Could you check a few things on this model? Use its own coordinates, in mm. A direction names the side the tool comes from. Round coordinates to 2 decimals unless told otherwise and drop trailing zeros. Write each loop counter-clockwise with the first axis right and the second up, starting at its lowest first coordinate (ties: lowest second). Pieces come first, ordered by that corner, then holes. Notation, with made-up numbers: M -33.75,-11.5 L -23.75,-11.5 A18 cw -23.75,16.5 Z; hole C 42.25,74.25 d6. An arc over 180 degrees is marked long. One line per item, written item: value. Start each with the question number.
(1) If I drill on L1, parallel to Y at x = 5.5, z = 5 (3 decimals); L2, parallel to X at y = -8.5, z = 10; L3, parallel to X at y = -4.25, z = -11, over which ranges is the centre line in solid material (lowest first)?
(2) Thinking about a two-plate mould opening in X: for faces 5 (the face through (0, -0.025, 19)), 6 (the face through (-13.157, -6, -22)), 7 (the face through (0, -3, 22.542)), 8 (the face through (0, -4.267, 22)), which applies, released by +X, released by -X, zero draft, split by the parting line, or undercut?
(3) I want a section at A-A on z = 8. Please give me the cut outline in (x, y) (1 decimal).
(4) Which directions (+Z, -Z, +X, -X, +Y, -Y) give clear straight access to the entire face, cutting with the end or side of a thin tool? Please do faces 1 (the face through (-5.4, -6.528, 21.9)), 2 (the face through (-10, -9.347, 22)), 3 (the face through (5.893, -8, 22)), 4 (the face through (-9, 0.203, -22)).
(5) I want a section at D-D on z = 20. Please give me the cut outline in (x, y), and give its area (3 significant figures).
(6) I want a section at C-C on y = -2.75. Count the separate pieces of the cut face and the enclosed holes in it, and give its area (3 significant figures).
(7) I'm going to push flat-ended pins straight in: pin 1 Ø1.5 at (y, z) = (-6.5, -19.5) entering from -X; pin 2 Ø1 at (x, z) = (1.5, -14.5) entering from -Y; pin 3 Ø5.5 at (y, z) = (-4.5, -19) entering from +X. Where does each tip first touch, or does it pass through?
```python
from build123d import *

# Parameters (mm, degrees)
BOSS_EXTRUDE1_DEPTH = 16.1925
SKETCH2_R           = 1.27
CUT_EXTRUDE1_DEPTH  = 5.08
BOSS_EXTRUDE2_DEPTH = 5.08
BOSS_EXTRUDE3_DEPTH = 1.27


with BuildPart() as part:
    # Sketch1 → Boss-Extrude1 (new body, symmetric)
    with BuildSketch(Plane.XY):
        Polygon((13.208, 0.254), (13.208, -9.398), (5.842, -9.398), (5.842, -6.985), (4.826, -6.985), (4.826, -6.477), (5.842, -6.477), (5.842, -4.318), (-5.842, -4.318), (-5.842, -6.477), (-4.826, -6.477), (-4.826, -6.985), (-5.842, -6.985), (-5.842, -9.398), (-13.208, -9.398), (-13.208, 0.254), (-7.367499011, 0.254), (-6.958302098, 0), (6.958302098, 0), (7.367499011, 0.254), align=None)
    extrude(amount=BOSS_EXTRUDE1_DEPTH, both=True)

    # Sketch2 → Cut-Extrude1 (cut)
    with BuildSketch(Plane(origin=(0, 0.254, 0), x_dir=(1, 0, 0), z_dir=(0, 1, 0))):
        with Locations((-10.287749506, 10.3505)):
            Circle(SKETCH2_R)
        with Locations((10.287749506, 10.3505)):
            Circle(SKETCH2_R)
        with Locations((10.287749506, -10.3505)):
            Circle(SKETCH2_R)
        with Locations((-10.287749506, -10.3505)):
            Circle(SKETCH2_R)
    extrude(amount=-CUT_EXTRUDE1_DEPTH, mode=Mode.SUBTRACT)

    # Sketch3 → Boss-Extrude2 (add)
    with BuildSketch(Plane.XY.offset(16.1925)):
        with BuildLine():
            Line((5.8674, -4.2926), (5.8674, -6.5024))
            Line((5.8674, -6.5024), (4.8514, -6.5024))
            Line((4.8514, -6.5024), (4.8514, -6.9596))
            Line((4.8514, -6.9596), (5.8674, -6.9596))
            Line((5.8674, -6.9596), (5.8674, -9.3726))
            Line((5.8674, -9.3726), (13.1826, -9.3726))
            Line((13.1826, -9.3726), (13.1826, -2.3114))
            ThreePointArc((13.1826, -2.3114), (12.438651224, -0.515348776), (10.6426, 0.2286))
            Line((10.6426, 0.2286), (7.37474135, 0.2286))
            Line((7.37474135, 0.2286), (6.965544437, -0.0254))
            Line((6.965544437, -0.0254), (-6.965544437, -0.0254))
            Line((-6.965544437, -0.0254), (-7.37474135, 0.2286))
            Line((-7.37474135, 0.2286), (-10.6426, 0.2286))
            ThreePointArc((-10.6426, 0.2286), (-12.438651224, -0.515348776), (-13.1826, -2.3114))
            Line((-13.1826, -2.3114), (-13.1826, -9.3726))
            Line((-13.1826, -9.3726), (-5.8674, -9.3726))
            Line((-5.8674, -9.3726), (-5.8674, -6.9596))
            Line((-5.8674, -6.9596), (-4.8514, -6.9596))
            Line((-4.8514, -6.9596), (-4.8514, -6.5024))
            Line((-4.8514, -6.5024), (-5.8674, -6.5024))
            Line((-5.8674, -6.5024), (-5.8674, -4.2926))
            Line((-5.8674, -4.2926), (5.8674, -4.2926))
        make_face()
    boss_extrude2 = extrude(amount=BOSS_EXTRUDE2_DEPTH)

    # Sketch5 → Boss-Extrude3 (add)
    with BuildSketch(Plane.XY.offset(21.2725)):
        with BuildLine():
            Line((13.1572, -9.3472), (13.1572, -2.3114))
            ThreePointArc((13.1572, -2.3114), (12.420690712, -0.533309288), (10.6426, 0.2032))
            Line((10.6426, 0.2032), (7.381983689, 0.2032))
            Line((7.381983689, 0.2032), (6.972786776, -0.0508))
            Line((6.972786776, -0.0508), (-6.972786776, -0.0508))
            Line((-6.972786776, -0.0508), (-7.381983689, 0.2032))
            Line((-7.381983689, 0.2032), (-10.6426, 0.2032))
            ThreePointArc((-10.6426, 0.2032), (-12.420690712, -0.533309288), (-13.1572, -2.3114))
            Line((-13.1572, -2.3114), (-13.1572, -9.3472))
            Line((-13.1572, -9.3472), (-5.8928, -9.3472))
            Line((-5.8928, -9.3472), (-5.8928, -6.9342))
            Line((-5.8928, -6.9342), (-4.8768, -6.9342))
            Line((-4.8768, -6.9342), (-4.8768, -6.5278))
            Line((-4.8768, -6.5278), (-5.8928, -6.5278))
            Line((-5.8928, -6.5278), (-5.8928, -4.2672))
            Line((-5.8928, -4.2672), (5.8928, -4.2672))
            Line((5.8928, -4.2672), (5.8928, -6.5278))
            Line((5.8928, -6.5278), (4.8768, -6.5278))
            Line((4.8768, -6.5278), (4.8768, -6.9342))
            Line((4.8768, -6.9342), (5.8928, -6.9342))
            Line((5.8928, -6.9342), (5.8928, -9.3472))
            Line((5.8928, -9.3472), (13.1572, -9.3472))
        make_face()
    boss_extrude3 = extrude(amount=BOSS_EXTRUDE3_DEPTH)

    # Mirror2: Boss-Extrude2, Boss-Extrude3 across plane
    add(boss_extrude2.mirror(Plane.XY))
    add(boss_extrude3.mirror(Plane.XY))


solid = part.part
```
Found:
1. L1: y = -6.985 to -6.477, -4.318 to 0
1. L2: x = -13.21 to -5.84, 5.84 to 13.21
1. L3: x = -13.21 to -11.38, -9.2 to 9.2, 11.38 to 13.21
2. face 5: undercut
2. face 6: released by -X
2. face 7: zero draft
2. face 8: undercut
3. outline: M -13.2,-9.4 L -5.8,-9.4 L -5.8,-7 L -4.8,-7 L -4.8,-6.5 L -5.8,-6.5 L -5.8,-4.3 L 5.8,-4.3 L 5.8,-6.5 L 4.8,-6.5 L 4.8,-7 L 5.8,-7 L 5.8,-9.4 L 13.2,-9.4 L 13.2,0.3 L 7.4,0.3 L 7,0 L -7,0 L -7.4,0.3 L -13.2,0.3 Z
4. face 1: +Z
4. face 2: +Z, +X, -X, -Y
4. face 3: +Z, -Y
4. face 4: -Z, +X, -X, +Y
5. outline: M -13.18,-9.37 L -5.87,-9.37 L -5.87,-6.96 L -4.85,-6.96 L -4.85,-6.5 L -5.87,-6.5 L -5.87,-4.29 L 5.87,-4.29 L 5.87,-6.5 L 4.85,-6.5 L 4.85,-6.96 L 5.87,-6.96 L 5.87,-9.37 L 13.18,-9.37 L 13.18,-2.31 A2.54 ccw 10.64,0.23 L 7.37,0.23 L 6.97,-0.03 L -6.97,-0.03 L -7.37,0.23 L -10.64,0.23 A2.54 ccw -13.18,-2.31 Z
5. area: 188 mm²
6. separate pieces: 1
6. enclosed holes: 4
6. area: 1,170 mm²
7. pin 1: stops at x = -13.18
7. pin 2: stops at y = -4.32
7. pin 3: stops at x = 13.18
